from build123d import *

# Parameters (mm, degrees)
SKETCH1_R           = 5
BOSS_EXTRUDE1_DEPTH = 50
BOSS_EXTRUDE2_DEPTH = 70
FILLET1_R           = 5
FILLET2_R           = 2
FILLET3_R           = 2
CHAMFER1_SIZE       = 3
CHAMFER1_SIZE2      = 5.196152423


# Some blends are built 0.0001 mm under size
with BuildPart() as part:
    # Sketch1 → Boss-Extrude1 (new body)
    with BuildSketch(Plane(origin=(0, 0, 0), x_dir=(1, 0, 0), z_dir=(0, 1, 0))):
        with Locations(Location((0, 0, 0), (0, 0, 270))):
            Circle(SKETCH1_R)
    extrude(amount=BOSS_EXTRUDE1_DEPTH)

    # Sketch2 → Boss-Extrude2 (add)
    with BuildSketch(Plane(origin=(0, 50, 0), x_dir=(1, 0, 0), z_dir=(0, 1, 0))):
        with BuildLine():
            Line((-5, 0), (-5, -30))
            Line((-5, -30), (5, -30))
            Line((5, -30), (5, 0))
            ThreePointArc((5, 0), (0, 5), (-5, 0))
        make_face()
    extrude(amount=BOSS_EXTRUDE2_DEPTH)

    # Fillet1
    fillet1_edges = [part.edges().sort_by_distance(p)[0] for p in [
        (-5, 85, 30),
        (5, 85, 30),
    ]]
    fillet(fillet1_edges, radius=FILLET1_R - 0.0001)  # a hair under: the kernel refuses the full size

    # Fillet2
    # the kernel refuses this fillet: 2 mm, written as the material it takes off along each edge
    with BuildSketch(Plane(origin=(5, 50, 25.0001), x_dir=(-1, 0, 0), z_dir=(0, 0, -1))) as fillet2_piece_1_section:
        with BuildLine():
            CenterArc((FILLET2_R, FILLET2_R), FILLET2_R, 180, 90)
            Line((0, FILLET2_R), (0, 0))
            Line((0, 0), (FILLET2_R, 0))
        make_face()
    fillet2_piece_1 = extrude(amount=30.0001, mode=Mode.PRIVATE)
    fillet2_piece_1 = fillet2_piece_1 - Plane(origin=(0, 50.338854102, 0), x_dir=(0, 0, 1), z_dir=(0, -1, 0)) * Cylinder(5, 69, mode=Mode.PRIVATE)
    add(fillet2_piece_1, mode=Mode.SUBTRACT)
    with BuildSketch(Plane(origin=(0.0001, 50, 25.0001), x_dir=(1, 0, 0), z_dir=(0, 0, -1))) as fillet2_piece_2:
        with BuildLine():
            CenterArc((4.9999 - FILLET2_R, -FILLET2_R), FILLET2_R, 0, 90)
            Line((4.9999, -FILLET2_R), (4.9999, 0))
            Line((4.9999, 0), (4.9999 - FILLET2_R, 0))
        make_face()
    revolve(axis=Axis((0.0001, 50, 25.0001), (0, -1, 0)), revolution_arc=90, mode=Mode.SUBTRACT)
    with BuildSketch(Plane(origin=(-0.0001, 50, 25.0001), x_dir=(0, 0, 1), z_dir=(1, 0, 0))) as fillet2_piece_3:
        with BuildLine():
            CenterArc((4.9999 - FILLET2_R, -FILLET2_R), FILLET2_R, 0, 90)
            Line((4.9999, -FILLET2_R), (4.9999, 0))
            Line((4.9999, 0), (4.9999 - FILLET2_R, 0))
        make_face()
    revolve(axis=Axis((-0.0001, 50, 25.0001), (0, -1, 0)), revolution_arc=90, mode=Mode.SUBTRACT)
    with BuildSketch(Plane(origin=(-5, 50, -5), x_dir=(1, 0, 0), z_dir=(0, 0, 1))) as fillet2_piece_4_section:
        with BuildLine():
            CenterArc((FILLET2_R, FILLET2_R), FILLET2_R, 180, 90)
            Line((0, FILLET2_R), (0, 0))
            Line((0, 0), (FILLET2_R, 0))
        make_face()
    fillet2_piece_4 = extrude(amount=30.0001, mode=Mode.PRIVATE)
    fillet2_piece_4 = fillet2_piece_4 - Plane(origin=(0, 50.465433579, 0), x_dir=(0, 0, 1), z_dir=(0, -1, 0)) * Cylinder(5, 69, mode=Mode.PRIVATE)
    add(fillet2_piece_4, mode=Mode.SUBTRACT)
    with BuildSketch(Plane(origin=(-0.0001, 50, 30), x_dir=(0, 0, -1), z_dir=(1, 0, 0))) as fillet2_piece_5:
        with BuildLine():
            CenterArc((FILLET2_R, FILLET2_R), FILLET2_R, 180, 90)
            Line((0, FILLET2_R), (0, 0))
            Line((0, 0), (FILLET2_R, 0))
        make_face()
    extrude(amount=0.0002, mode=Mode.SUBTRACT)

    # Fillet3
    fillet3_edges = [part.edges().sort_by_distance(p)[0] for p in [
        (0, 0, -5),
    ]]
    fillet(fillet3_edges, radius=FILLET3_R)

    # Chamfer1
    chamfer1_edges = [part.edges().sort_by_distance(p)[0] for p in [
        (5, 120, 12.50005),
        (3.535563195, 120, 28.535563195),
        (-3.535563195, 120, 28.535563195),
        (0, 120, -5),
        (-5, 120, 12.50005),
    ]]
    chamfer1_side = [part.faces().sort_by_distance(p)[0] for p in [
        (0, 120, 12.500020673),
    ]]
    chamfer(chamfer1_edges, length=CHAMFER1_SIZE, length2=CHAMFER1_SIZE2, reference=chamfer1_side[0])


solid = part.part
Input: part model. Units: mm. Frame: model coordinates. A direction names the side the tool comes from. Give positions to 0.01 mm unless a question says otherwise; leave off trailing zeros. Order: outer loops, then holes, each group sorted by start corner. A loop starts at its lowest first (then second) coordinate and runs counter-clockwise, first axis right, second up.
Q1. Section A-A on z = 10. Output: boundary loops of the cut face in (x, y), and give its area (3 significant figures).
Checked values:
outline: (-5, 52) arc R2 ccw to (-3, 50) - (3, 50) arc R2 ccw to (5, 52) - (5, 114.8) - (2, 120) - (-2, 120) - (-5, 114.8) - close
area: 683 mm2
Q2. Section C-C on y = 38. Output: boundary loops of the cut face in (x, z), and give its area (3 significant figures).
Checked values:
outline: circle Ø10 at (0, 0)
area: 78.5 mm2
Q3. Contact query for flat-ended pins moving along their axis: pin 1 Ø1.5 at (x, y) = (0.5, 69.5) entering from -Z; pin 2 Ø5 at (x, z) = (3, 23.5) entering from -Y. Output: stop coordinate, or through.
Checked values:
pin 1: stops at z = -5
pin 2: stops at y = 50
Q4. Set-up query: faces 1 (the cylindrical face through (4.43, 50.6, 12.68)), 2 (the cylindrical face through (-4.43, 50.6, 12.33)), 3 (the conical face through (-2.517, 117.366, 27.462)). Return all of +Z, -Z, +X, -X, +Y, -Y with unobstructed straight access to the full face (end or side cutting, diameter ignored); none if empty.
Checked values:
face 1: +Z, +X, -Y
face 2: +Z, -X, -Y
face 3: +Z, -X, +Y
Q5. Ray query, probe 1 along Y at (x, z) = (0.5, 17.5); probe 2 along Z at (x, y) = (4, 48.5); probe 3 along Z at (x, y) = (1.5, 73). Return the intervals inside material, ascending.
Checked values:
probe 1: y = 50 to 120
probe 2: z = -3 to 3
probe 3: z = -4.77 to 29.77
